```python
from build123d import *

# Parameters (mm, degrees)
ESQUISSE1_W                                        = 25
ESQUISSE1_H                                        = 58
BOSS_EXTRU_1_DEPTH                                 = 10
ESQUISSE3_R                                        = 10
ENL_V_MAT_EXTRU_2_DEPTH                            = 5
ESQUISSE4_R                                        = 6.25
ENL_V_MAT_EXTRU_3_DEPTH                            = 6
CHAMBRAGE_POUR_VIS_T_TE_HEXAGONALE_M51_D           = 5.5
CHAMBRAGE_POUR_VIS_T_TE_HEXAGONALE_M51_CBORE_D     = 10
CHAMBRAGE_POUR_VIS_T_TE_HEXAGONALE_M51_CBORE_DEPTH = 5
CHAMBRAGE_POUR_VIS_T_TE_HEXAGONALE_M53_D           = 5.5
CHAMBRAGE_POUR_VIS_T_TE_HEXAGONALE_M53_CBORE_D     = 10
CHAMBRAGE_POUR_VIS_T_TE_HEXAGONALE_M53_CBORE_DEPTH = 5
TROU_TARAUD_M43_D                                  = 3.3
TROU_TARAUD_M42_D                                  = 3.3


with BuildPart() as part:
    # Esquisse1 → Boss.-Extru.1 (new body)
    with BuildSketch(Plane.XY):
        Rectangle(ESQUISSE1_W, ESQUISSE1_H)
    extrude(amount=BOSS_EXTRU_1_DEPTH)

    # Esquisse3 → Enlèv. mat.-Extru.2 (cut)
    with BuildSketch(Plane(origin=(0, 0, 0), x_dir=(-1, 0, 0), z_dir=(0, 0, -1))):
        Circle(ESQUISSE3_R)
    extrude(amount=-ENL_V_MAT_EXTRU_2_DEPTH, mode=Mode.SUBTRACT)

    # Esquisse4 → Enlèv. mat.-Extru.3 (cut, through all)
    with BuildSketch(Plane(origin=(0, 0, 5), x_dir=(-1, 0, 0), z_dir=(0, 0, -1))):
        Circle(ESQUISSE4_R)
    extrude(amount=-ENL_V_MAT_EXTRU_3_DEPTH, mode=Mode.SUBTRACT)

    # Chambrage pour vis à tête hexagonale M51 (through all)
    with Locations(Plane.XY.offset(10)):
        with Locations((0, -20)):
            CounterBoreHole(CHAMBRAGE_POUR_VIS_T_TE_HEXAGONALE_M51_D / 2, CHAMBRAGE_POUR_VIS_T_TE_HEXAGONALE_M51_CBORE_D / 2, CHAMBRAGE_POUR_VIS_T_TE_HEXAGONALE_M51_CBORE_DEPTH)

    # Chambrage pour vis à tête hexagonale M53 (through all)
    with Locations(Plane.XY.offset(10)):
        with Locations((0, 20)):
            CounterBoreHole(CHAMBRAGE_POUR_VIS_T_TE_HEXAGONALE_M53_D / 2, CHAMBRAGE_POUR_VIS_T_TE_HEXAGONALE_M53_CBORE_D / 2, CHAMBRAGE_POUR_VIS_T_TE_HEXAGONALE_M53_CBORE_DEPTH)

    # Trou taraudé M43 (through all)
    with Locations(Plane(origin=(12.5, 0, 0), x_dir=(0, 0, -1), z_dir=(1, 0, 0))):
        with Locations((-5, 12)):
            Hole(TROU_TARAUD_M43_D / 2)

    # Trou taraudé M42 (through all)
    with Locations(Plane.ZY.offset(12.5)):
        with Locations((5, -12)):
            Hole(TROU_TARAUD_M42_D / 2)


solid = part.part
```
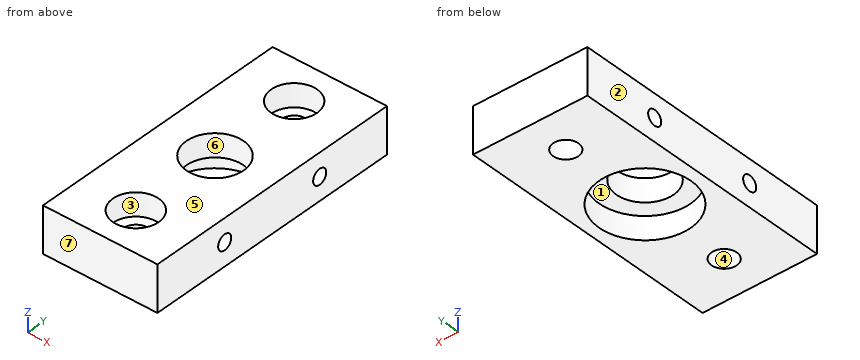
CAD build for the part. Positions are in the model's coordinates, mm. Face numbers are marked on the shaded views. A direction names the side the tool comes from. Round coordinates to 2 decimals unless told otherwise and drop trailing zeros. Order: outer loops, then holes, each group sorted by start corner. A loop starts at its lowest first (then second) coordinate and runs counter-clockwise, first axis right, second up.
Item 1: Saw through at C-C on y = 8. Write the cut outline in (x, z).
Item 2: Tool access for the marked faces 1, 2 and 3: list every direction of +Z, -Z, +X, -X, +Y, -Y with a clear straight run to the whole face (end or side of a thin tool).
Item 3: Saw through at A-A on y = -12. Write the cut outline in (x, z).
Item 4: Probe line 1 along Y through (x, z) = (0, 9); line 2 along Y through (x, z) = (-4.25, 6.75); line 3 along Y through (x, z) = (0, 3.65). List the from-to ranges inside material, lowest first.
Item 5: Mould opens along Y. For the marked faces 4, 5, 6 and 7 say: pulls with the +Y half, pulls with the -Y half, needs draft (parallel to the pull), parting line crosses it, or undercut.
Item 6: Pin check, flat tips, straight feed: pin 1 (3 mm diameter, centred on x = -2, y = -19, fed in from +Z); pin 2 (6 mm diameter, centred on x = -4.5, y = 1, fed in from -Z). Stop position of each tip, or through.
Item 7: Saw through at B-B on x = -7.75. Write the cut outline in (y, z).
Item 8: Saw through at D-D on y = -20. Write the cut outline in (x, z), then the cut area to 4 significant figures.
Reported:
1. outline: (-12.5, 0) - (-6, 0) - (-6, 5) - (6, 5) - (6, 0) - (12.5, 0) - (12.5, 10) - (-12.5, 10) - close
2. face 1: -Z
2. face 2: +Z, -Z, -X, +Y, -Y
2. face 3: +Z
3. outline: (-12.5, 0) - (12.5, 0) - (12.5, 3.35) - (-12.5, 3.35) - close; (-12.5, 6.65) - (12.5, 6.65) - (12.5, 10) - (-12.5, 10) - close
4. line 1: y = -29 to -25, -15 to -6.25, 6.25 to 15, 25 to 29
4. line 2: y = -29 to -22.63, -17.37 to -4.58, 4.58 to 17.37, 22.63 to 29
4. line 3: y = -29 to -22.75, -17.25 to -12.95, -11.05 to -10, 10 to 11.05, 12.95 to 17.25, 22.75 to 29
5. face 4: undercut
5. face 5: needs draft
5. face 6: undercut
5. face 7: pulls with the -Y half
6. pin 1: stops at z = 5
6. pin 2: stops at z = 5
7. outline: (-29, 0) - (-6.32, 0) - (-6.32, 5) - (6.32, 5) - (6.32, 0) - (29, 0) - (29, 10) - (-29, 10) - close; hole circle Ø3.3 at (-12, 5); hole circle Ø3.3 at (12, 5)
8. outline: (-12.5, 0) - (-2.75, 0) - (-2.75, 5) - (-5, 5) - (-5, 10) - (-12.5, 10) - close; (2.75, 0) - (12.5, 0) - (12.5, 10) - (5, 10) - (5, 5) - (2.75, 5) - close
8. area: 172.5 mm2
